For this review, take the finished solid that the model builds, in its own axes (mm). A direction names the side the tool comes from. Give positions to 0.01 mm unless a question says otherwise; leave off trailing zeros. Write each loop counter-clockwise with the first axis right and the second up, starting at its lowest first coordinate (ties: lowest second). Pieces come first, ordered by that corner, then holes.
1) For P1, Ø1.8, axis at x = 25, z = 3, coming from the +Y side; P2, Ø3, axis at x = 15, z = 4, coming from the -Y side, all flat-tipped, find the tip position at first contact; note any pin that passes through.
2) Draft analysis for pull direction X (two halves, no side actions). For faces 1 (the face through (38.91, -14.84, 2.96)), 2 (the face through (-30, -163, 3)), 3 (the face through (-86.5, 2, 3)), state which applies: pulls with the +X half, pulls with the -X half, needs draft (parallel to the pull), parting line crosses it, or undercut.
3) Machinability: for faces 4 (the face through (86.5, 38, 3)), 5 (the face through (41, 155, 3)), which of the approach directions +Z, -Z, +X, -X, +Y, -Y give a long, thin tool a straight path to every point of the face, cutting with its end or side? Answer none if there is none.
4) We need section D-D on y = -6. Give the boundary of the cut face in (x, z), and give its area (3 significant figures).
5) Wall thickness on line 1 along Y through (x, z) = (46.5, 1.55); line 2 along Y through (x, z) = (49.5, 2.6); line 3 along X through (y, z) = (-10, 2.8): over which ranges is each line inside the solid? List them lowest first.
6) We need section C-C on x = 46.5. Give the boundary of the cut face in (y, z).
7) We need section B-B on z = 5. Give the boundary of the cut face in (x, y).
8) We need section A-A on y = 50. Give the boundary of the cut face in (x, z), and give its area (3 significant figures).
Autodesk Fusion 360 part; units mm, degrees
sketch "スケッチ1" plane through (0, 0, 0) normal (0, 0, 1) x (1, 0, 0)
  line L0 (-3.5, 163) -> (-86.5, 163)
  line L1 (-86.5, 163) -> (-86.5, -163)
  line L2 (-86.5, -163) -> (-3.5, -163)
  line L3 (86.5, -75) -> (86.5, 155)
  line L4 (82.2546, 155) -> (-86.5, -163) construction
  line L5 (-86.5, 163) -> (55.7541, -105.0627) construction
  line L6 (-3.5, 163) -> (-3.5, 155)
  line L7 (-3.5, 155) -> (86.5, 155)
  line L8 (-86.5, -163) -> (-3.5, -163) construction
  line L9 (86.5, -75) -> (-3.5, -163)
  dimension "d2" = 326
  dimension "d5" = 83
extrude "押し出し1" add sketch "スケッチ1" along normal blind 6
chamfer "面取り1" distance 30 angle 45 2 edges at (-86.5, -163, 3) (-86.5, 163, 3)
sketch "スケッチ2" plane through (0, 0, 6) normal (0, 0, 1) x (-1, 0, 0)
  line L0 (56.5, -163) -> (86.5, -133)
  line L1 (86.5, -133) -> (86.5, 133)
  line L2 (86.5, 133) -> (56.5, 163)
  line L3 (56.5, 163) -> (3.5, 163)
  line L4 (3.5, 163) -> (-86.5, 75)
  line L5 (-86.5, 75) -> (-86.5, -155)
  line L6 (-86.5, -155) -> (3.5, -155)
  line L7 (3.5, -155) -> (3.5, -163)
  line L8 (3.5, -163) -> (56.5, -163)
  line L9 (-86.5, -155) -> (-46.5, -155) construction
  line L10 (-46.5, -155) -> (-46.5, -110) construction
  line L11 (-46.5, -110) -> (-86.5, -110) construction
  line L12 (-86.5, -110) -> (-86.5, -155) construction
  line L13 (-46.5, -110) -> (-46.5, -50) construction
  line L14 (-46.5, -50) -> (-46.5, 10) construction
  point P0 (-46.5, -110)
  point P1 (-46.5, -50)
  point P2 (-46.5, 10)
  dimension "d10" = 40
  dimension "d11" = 45
  dimension "d12" = 60
  dimension "d13" = 60
hole "穴1" at (46.5, 110, 6) at (46.5, 50, 6) at (46.5, -10, 6) direction (0, 0, -1) diameter 18 end through all
equation "d5 = 30 mm + 53 mm"
Results list:
1. P1: stops at y = 155
1. P2: stops at y = -146.38
2. face 1: undercut
2. face 2: needs draft
2. face 3: pulls with the -X half
3. face 4: +Z, -Z, +X, +Y, -Y
3. face 5: +Z, -Z, +X, +Y
4. outline: (-86.5, 0) - (38.44, 0) - (38.44, 6) - (-86.5, 6) - close; (54.56, 0) - (86.5, 0) - (86.5, 6) - (54.56, 6) - close
4. area: 941 mm2
5. line 1: y = -114.11 to -19, -1 to 41, 59 to 101, 119 to 155
5. line 2: y = -111.18 to -18.49, -1.51 to 41.51, 58.49 to 101.51, 118.49 to 155
5. line 3: x = -86.5 to 37.5, 55.5 to 86.5
6. outline: (-114.11, 0) - (-19, 0) - (-19, 6) - (-114.11, 6) - close; (-1, 0) - (41, 0) - (41, 6) - (-1, 6) - close; (59, 0) - (101, 0) - (101, 6) - (59, 6) - close; (119, 0) - (155, 0) - (155, 6) - (119, 6) - close
7. outline: (-86.5, -133) - (-56.5, -163) - (-3.5, -163) - (86.5, -75) - (86.5, 155) - (-3.5, 155) - (-3.5, 163) - (-56.5, 163) - (-86.5, 133) - close; hole circle Ø18 at (46.5, -10); hole circle Ø18 at (46.5, 50); hole circle Ø18 at (46.5, 110)
8. outline: (-86.5, 0) - (37.5, 0) - (37.5, 6) - (-86.5, 6) - close; (55.5, 0) - (86.5, 0) - (86.5, 6) - (55.5, 6) - close
8. area: 930 mm2
